Here's how the part is built. I have some questions about the finished solid (model axes, mm). A direction names the side the tool comes from. Give positions to 0.01 mm unless a question says otherwise; leave off trailing zeros. Order: outer loops, then holes, each group sorted by start corner. A loop starts at its lowest first (then second) coordinate and runs counter-clockwise, first axis right, second up. Notation, with made-up numbers: M -37.75,72 L 9.25,72 A23 cw 9.25,96 Z; hole C -40,5.25 d4. An arc over 180 degrees is marked long. One line per item, written item: value. Start each with the question number.
from build123d import *

# Parameters (mm, degrees)
SKETCH2_W           = 124.173
SKETCH2_H           = 119.38
BOSS_EXTRUDE1_DEPTH = 3.175
SKETCH4_R           = 1.905
SKETCH4_R_2         = 1.46
SKETCH4_W           = 86.3
SKETCH4_H           = 45.7
SKETCH4_W_2         = 61.5
SKETCH4_H_2         = 11.2
CUT_EXTRUDE1_DEPTH  = 14.175
SKETCH10_W          = 1.59
SKETCH10_H          = 120
CUT_EXTRUDE3_DEPTH  = 10
SKETCH11_R          = 1.905
CUT_EXTRUDE4_DEPTH  = 10


with BuildPart() as part:
    # Sketch2 → Boss-Extrude1 (new body)
    with BuildSketch(Plane.XY):
        with Locations((40.767155738, -50.87039032)):
            Rectangle(SKETCH2_W, SKETCH2_H)
    extrude(amount=BOSS_EXTRUDE1_DEPTH)

    # Sketch4 → Cut-Extrude1 (cut)
    with BuildSketch(Plane.XY):
        with Locations((-15.867344262, -37.32039032)):
            Circle(SKETCH4_R)
        with Locations((-15.867344262, -64.42239032)):
            Circle(SKETCH4_R)
        with Locations((79.302655738, 3.36760968)):
            Circle(SKETCH4_R)
        with Locations((79.300655738, -105.10839032)):
            Circle(SKETCH4_R)
        with Locations((64.353655738, -53.29939032)):
            Circle(SKETCH4_R_2)
        with Locations((64.353655738, -84.64939032)):
            Circle(SKETCH4_R_2)
        with Locations((30.720655738, -22.92039032)):
            Rectangle(SKETCH4_W, SKETCH4_H)
        with Locations((72.103655738, -69.11339032)):
            Rectangle(SKETCH4_W_2, SKETCH4_H_2)
    extrude(amount=CUT_EXTRUDE1_DEPTH, mode=Mode.SUBTRACT)

    # Sketch10 → Cut-Extrude3 (cut)
    with BuildSketch(Plane(origin=(102.853655738, 0, 0), x_dir=(0, 0, -1), z_dir=(1, 0, 0))):
        with Locations((-2.380000064, -51.180389625)):
            Rectangle(SKETCH10_W, SKETCH10_H)
    extrude(amount=-CUT_EXTRUDE3_DEPTH, mode=Mode.SUBTRACT)

    # Sketch11 → Cut-Extrude4 (cut)
    with BuildSketch(Plane.XY.offset(3.175)):
        with Locations((97.853655738, -9.262889625)):
            Circle(SKETCH11_R)
        with Locations((97.853655738, -27.345389625)):
            Circle(SKETCH11_R)
        with Locations((97.853655738, -45.43089032)):
            Circle(SKETCH11_R)
        with Locations((97.853655738, -96.56039032)):
            Circle(SKETCH11_R)
    extrude(amount=-CUT_EXTRUDE4_DEPTH, mode=Mode.SUBTRACT)


solid = part.part
Item 1: Will these pins go through, and if not, where does the flat tip stop? P1, Ø2.5, axis at x = -15.87, y = -64.42, coming from the -Z side; P2, Ø0.5, axis at y = -10.5, z = 2.5, coming from the +X side.
Item 2: I want a section at C-C on z = 0.65. Count the separate pieces of the cut face and the enclosed holes in it, plus the area to 3 significant figures.
Item 3: We'd pull the mould along Y, two halves only. Please class faces 1 (the face through (100, -28, 1.585)), 2 (the face through (-12.429, -23, 2)): +Y half, -Y half, draft (parallel to the pull), parting line (faces both ways), or undercut.
Item 4: I want a section at A-A on x = 39. Write out the boundary of the cut face in (y, z) (3 decimals).
Item 5: I want a section at B-B on y = -16. Write out the boundary of the cut face in (x, z) (3 decimals), plus the area to 3 significant figures.
Item 6: I want a section at D-D on x = 56. Write out the boundary of the cut face in (y, z) (3 decimals).
Item 7: Please list where these lines run through material, in increasing order: probe 1 along Y at (x, z) = (53.5, 1.85); probe 2 along Y at (x, z) = (26.5, 2.65); probe 3 along Y at (x, z) = (77, 2.3). Write a range as [from, to].
Item 8: For faces 3 (the face through (98, -93, 1.585)), 4 (the face through (72, -74.713, 2)), 5 (the face through (-21.319, -52, 2)), 6 (the face through (30, -0.07, 2)), which set-ups out of +Z, -Z, +X, -X, +Y, -Y let a thin tool reach every point of the face, with its end or its side?
Answer below:
1. P1: passes through
1. P2: stops at x = 92.85
2. separate pieces: 1
2. enclosed holes: 11
2. area: 10,100 mm²
3. face 1: draft
3. face 2: undercut
4. outline: M -110.56,0 L -45.77,0 L -45.77,3.175 L -110.56,3.175 Z; M -0.07,0 L 8.82,0 L 8.82,3.175 L -0.07,3.175 Z
5. outline: M -21.319,0 L -12.429,0 L -12.429,3.175 L -21.319,3.175 Z; M 73.871,0 L 102.854,0 L 102.854,1.585 L 92.854,1.585 L 92.854,3.175 L 73.871,3.175 Z
5. area: 104 mm²
6. outline: M -110.56,0 L -74.713,0 L -74.713,3.175 L -110.56,3.175 Z; M -63.513,0 L -45.77,0 L -45.77,3.175 L -63.513,3.175 Z; M -0.07,0 L 8.82,0 L 8.82,3.175 L -0.07,3.175 Z
7. probe 1: y = [-110.56, -74.71], [-63.51, -45.77], [-0.07, 8.82]
7. probe 2: y = [-110.56, -45.77], [-0.07, 8.82]
7. probe 3: y = [-110.56, -74.71], [-63.51, 8.82]
8. face 3: +Z, +X, +Y, -Y
8. face 4: +Z, -Z, +X
8. face 5: +Z, -Z, -X, +Y, -Y
8. face 6: +Z, -Z
